Work out the finished part from the listing and answer in its coordinate system (mm). Face numbers are marked on the shaded views. A direction names the side the tool comes from. Give positions to 0.01 mm unless a question says otherwise; leave off trailing zeros. Order: outer loops, then holes, each group sorted by start corner. A loop starts at its lowest first (then second) coordinate and runs counter-clockwise, first axis right, second up. Notation, with made-up numbers: (37, -4) - (56, -4) arc R17 cw to (56, 18) - close; hole circle Ø11 at (49, 74.25). An arc over 180 degrees is marked (long way). Write each question's results on one line, items separated by ' | '.
from build123d import *

# Parameters (mm, degrees)
RESSALTO_EXTRUS_O1_DEPTH = 7.5
ESBO_O2_R                = 1.7500000000000029
CORTE_EXTRUS_O1_DEPTH    = 10
FILETE1_R                = 1
CORTE_EXTRUS_O2_START    = -5
CORTE_EXTRUS_O2_DEPTH    = 75
FILETE2_R                = 3
FILETE3_R                = 8
FILETE4_R                = 4


with BuildPart() as part:
    # Esboço1 → Ressalto-extrusão1 (new, symmetric)
    with BuildSketch(Plane.XY):
        Polygon((-2.4999999999999947, -2.5000000000002314), (-77.5, -2.5000000000002305), (-77.5, 5.499999999999769), (-82.5, 5.499999999999769), (-82.5, -2.5000000000002314), (-82.5, -13.4491378645859), (-2.499999999999993, -32.50000000000023), (-2.499999999999994, -97.5000000000002), (2.500000000000006, -97.50000000000021), (2.4999999999999813, 97.4999999999998), (-2.4999999999999933, 97.4999999999998), align=None)
        Polygon((-2.4999999999999947, -9.500000000000231), (-25.833333333333332, -9.500000000000231), (-25.833333333333332, -21.80368179578865), (-2.499999999999992, -27.360183251951156), align=None, mode=Mode.SUBTRACT)
        Polygon((-77.5, -9.500000000000231), (-30.83333333333334, -20.613002912325253), (-30.833333333333336, -9.500000000000231), align=None, mode=Mode.SUBTRACT)
    extrude(amount=RESSALTO_EXTRUS_O1_DEPTH, both=True)

    # Esboço2 → Corte-extrusão1 (cut)
    with BuildSketch(Plane.ZY.offset(2.4999999999999947)):
        with Locations(Location((0, 90, 0), (0, 0, 270))):
            Circle(ESBO_O2_R)
        with Locations(Location((0, -90, 0), (0, 0, 270))):
            Circle(ESBO_O2_R)
    extrude(amount=-CORTE_EXTRUS_O1_DEPTH, mode=Mode.SUBTRACT)

    # Filete1
    filete1_edges = [part.edges().sort_by_distance(p)[0] for p in [
        (-77.5, -9.500000000000231, 0),
    ]]
    fillet(filete1_edges, radius=FILETE1_R)

    # Esboço3 → Corte-extrusão2 (cut)
    with BuildSketch(Plane.ZY.offset(82.5).offset(CORTE_EXTRUS_O2_START)):
        with BuildLine():
            Line((7.5, -4.5096189432336615), (7.5, -2.5000000000002363))
            Line((7.5, -2.5000000000002363), (0, -2.5000000000002363))
            ThreePointArc((-4.4e-16, -2.50000000000024), (3.8822856765378098, -3.0111126056642163), (7.500000000000002, -4.509618943233658))
        make_face()
        with BuildLine():
            ThreePointArc((-7.500000000000002, -4.509618943233658), (-3.8822856765378124, -3.0111126056642163), (-4.4e-16, -2.50000000000024))
            Line((0, -2.5000000000002363), (-7.5, -2.5000000000002363))
            Line((-7.5, -2.5000000000002363), (-7.5, -4.5096189432336615))
        make_face()
    extrude(amount=-CORTE_EXTRUS_O2_DEPTH, mode=Mode.SUBTRACT)

    # Filete2
    filete2_edges = [part.edges().sort_by_distance(p)[0] for p in [
        (-6.22e-15, 97.4999999999998, -7.5),
        (6.22e-15, -97.5000000000002, -7.5),
        (-6.22e-15, 97.4999999999998, 7.5),
        (6.22e-15, -97.5000000000002, 7.5),
    ]]
    fillet(filete2_edges, radius=FILETE2_R)

    # Filete3
    filete3_edges = [part.edges().sort_by_distance(p)[0] for p in [
        (-2.499999999999993, -32.50000000000023, 0),
        (-82.5, -13.4491378645859, 0),
    ]]
    fillet(filete3_edges, radius=FILETE3_R)

    # Filete4
    filete4_edges = [part.edges().sort_by_distance(p)[0] for p in [
        (-77.5, -2.5000000000002327, -1.44e-15),
    ]]
    fillet(filete4_edges, radius=FILETE4_R)


solid = part.part
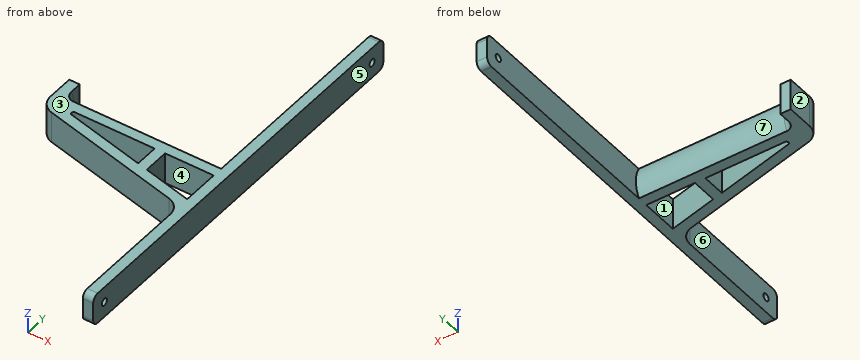
1. Determine the mould class of the marked faces 1, 2 and 3 for opening direction X: +X half, -X half, draft (parallel to the pull), parting line (faces both ways), or undercut.
Answer list:
face 1: undercut | face 2: -X half | face 3: draft
2. Given P1, Ø7.5, axis at x = -18.5, z = -0.5, coming from the -Y side; P2, Ø1.5, axis at x = -23, z = 2.5, coming from the +Y side; P3, Ø4, axis at x = -80, z = 0, coming from the +Y side; P4, Ø12, axis at x = -31, y = -27.5, coming from the -Z side, each flat-ended and moving along its own axis, determine where each tip first touches the part or whether it passes through.
Answer list:
P1: y = -29.58 | P2: y = -2.6 | P3: y = 5.5 | P4: z = -7.5
3. A cutting plane is placed at B-B, the plane z = 0. State how many separate pieces and enclosed holes the cut face has, then the cut area to 3 significant figures.
Answer list:
separate pieces: 3 | enclosed holes: 2 | area: 2,020 mm^2
4. A tool of negligible diameter and unlimited length cuts with its end or side. For the marked faces 4, 5, 6 and 7, from which of +Z, -Z, +X, -X, +Y, -Y can it reach the whole face along a straight path? Write none if from no direction.
Answer list:
face 4: +Z, -Z | face 5: +Z, -Z, +X, +Y, -Y | face 6: +Z, -Z, -X, -Y | face 7: +Y
5. Straight lines are drawn through the part: line 1 (X direction, y = 1.5, z = 7); line 2 (Z direction, x = -0.35, y = -90); line 3 (X direction, y = 25, z = -3.75). For each, find the intervals that lie inside material, in ascending order. Write a range as [from, to].
Answer list:
line 1: [-82.5, -77.5], [-2.5, 2.5] | line 2: [-7.5, -1.75], [1.75, 7.5] | line 3: [-2.5, 2.5]
6. A cutting plane is placed at D-D, the plane y = -56. Write down the section's boundary in (x, z).
Answer list:
outline: (-2.5, -7.5) - (2.5, -7.5) - (2.5, 7.5) - (-2.5, 7.5) - close
7. A cutting plane is placed at C-C, the plane x = -12. Write down the section's boundary in (y, z).
Answer list:
outline: (-30.24, -7.5) - (-25.1, -7.5) - (-25.1, 7.5) - (-30.24, 7.5) - close; (-9.5, -7.5) - (-4.51, -7.5) arc R15 ccw to (-4.51, 7.5) - (-9.5, 7.5) - close
8. A cutting plane is placed at A-A, the plane y = -90. Write down the section's boundary in (x, z).
Answer list:
outline: (-2.5, -7.5) - (2.5, -7.5) - (2.5, -1.75) - (-2.5, -1.75) - close; (-2.5, 1.75) - (2.5, 1.75) - (2.5, 7.5) - (-2.5, 7.5) - close
